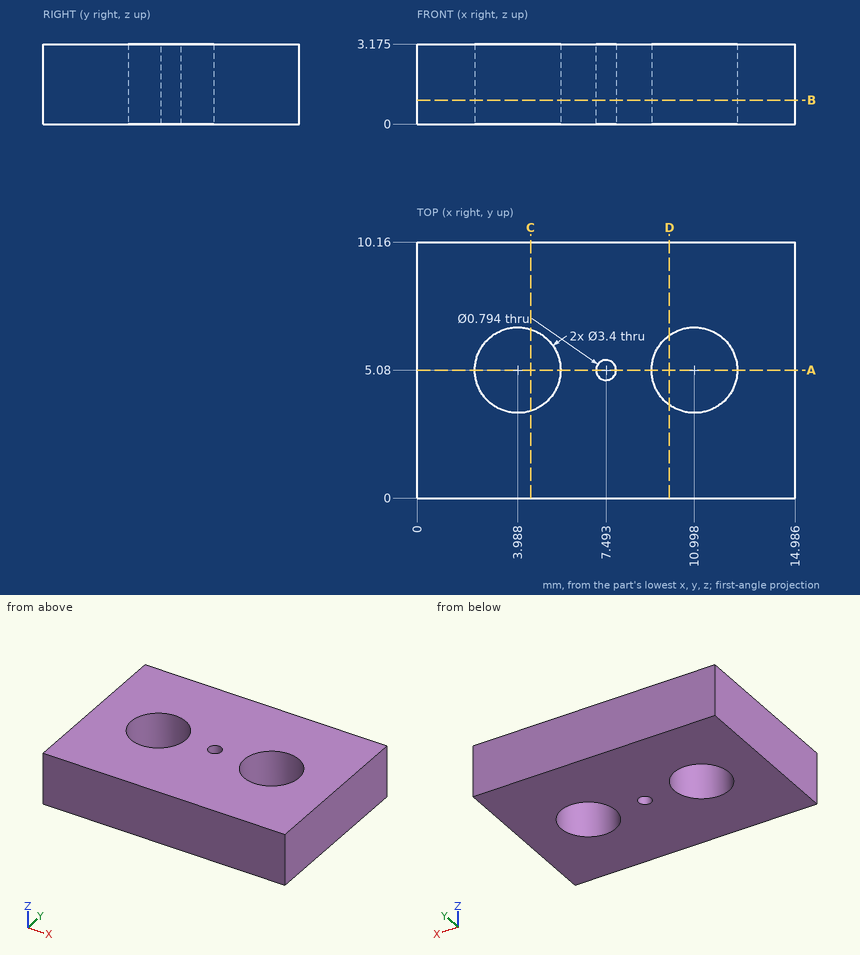
Geometry check sheet. Reference: drawing and pictorial views, mm from the part's lowest x, y, z. Coordinates: 2 decimals unless noted, no trailing zeros. Order: outer loops, then holes, each group sorted by start corner. A loop starts at its lowest first (then second) coordinate and runs counter-clockwise, first axis right, second up. Notation, with made-up numbers: (26.5, 24.25) -> (36.5, 24.25) arc R14 ccw to (36.5, 50.25) -> close; hole circle Ø1 at (41, 24). An arc over 180 degrees is marked (long way). Use CSV: the item, a comma, the result in double quotes. Start each with the question number.
Q1. Section check B-B, the plane z = 0.95. Record the cut outline in (x, y), and give its area (3 significant figures).
Q2. Thickness scan on line 1 along X through (y, z) = (4.75, 2.2) (1 decimal); line 2 along Y through (x, z) = (7.5, 2.7); line 3 along X through (y, z) = (4, 0.8) (1 decimal). Record the ranges inside material, lowest first.
Q3. Section check D-D, the plane x = 10. Record the cut outline in (y, z) (1 decimal).
Q4. Section check C-C, the plane x = 4.5. Record the cut outline in (y, z) (1 decimal), and give its area (3 significant figures).
Q5. Depth check by flat-ended pin: P1, Ø2, axis at x = 3.99, y = 5.08, coming from the +Z side (3 decimals). Enter the tip coordinate at first touch or a pass-through.
Q6. Section check A-A, the plane y = 5.08. Record the cut outline in (x, z) (1 decimal).
Returned:
1,outline,"(0, 0) -> (14.99, 0) -> (14.99, 10.16) -> (0, 10.16) -> close; hole circle Ø3.4 at (3.99, 5.08); hole circle Ø0.79 at (7.49, 5.08); hole circle Ø3.4 at (11, 5.08)"
1,area,"134 mm^2"
2,line 1,"x = 0 to 2.3, 5.7 to 7.3, 7.7 to 9.3, 12.7 to 15"
2,line 2,"y = 0 to 4.68, 5.48 to 10.16"
2,line 3,"x = 0 to 2.7, 5.3 to 9.7, 12.3 to 15"
3,outline,"(0, 0) -> (3.7, 0) -> (3.7, 3.2) -> (0, 3.2) -> close; (6.5, 0) -> (10.2, 0) -> (10.2, 3.2) -> (6.5, 3.2) -> close"
4,outline,"(0, 0) -> (3.5, 0) -> (3.5, 3.2) -> (0, 3.2) -> close; (6.7, 0) -> (10.2, 0) -> (10.2, 3.2) -> (6.7, 3.2) -> close"
4,area,"22.0 mm^2"
5,P1,"passes through"
6,outline,"(0, 0) -> (2.3, 0) -> (2.3, 3.2) -> (0, 3.2) -> close; (5.7, 0) -> (7.1, 0) -> (7.1, 3.2) -> (5.7, 3.2) -> close; (7.9, 0) -> (9.3, 0) -> (9.3, 3.2) -> (7.9, 3.2) -> close; (12.7, 0) -> (15, 0) -> (15, 3.2) -> (12.7, 3.2) -> close"
